Geometry check sheet. Reference: the model listing, model coordinates, mm. Give positions to 0.01 mm unless a question says otherwise; leave off trailing zeros. Write each loop counter-clockwise with the first axis right and the second up, starting at its lowest first coordinate (ties: lowest second). Pieces come first, ordered by that corner, then holes. Notation, with made-up numbers: (1.25, 84.25) -> (23.25, 84.25) arc R19 cw to (23.25, 121.25) -> close; hole circle Ø10 at (2.5, 10.5). An arc over 180 degrees is marked (long way). Write item = value, one per line. Start each with the question number.
1. Thickness scan on line 1 along Z through (x, y) = (27, 96.5); line 2 along X through (y, z) = (48, -7); line 3 along Y through (x, z) = (1, -5). Record the ranges inside material, lowest first.
2. Cross-section at C-C, the plane z = -7.75. Record the cut outline in (x, y) (3 decimals), plus the area to 3 significant figures.
3. Cross-section at B-B, the plane y = 13. Record the cut outline in (x, z), plus the area to 3 significant figures.
4. Cross-section at A-A, the plane x = 59. Record the cut outline in (y, z) (3 decimals).
5. Depth check by flat-ended pin: P1, Ø5, axis at x = 12, z = -10, coming from the +Y side; P2, Ø2.5, axis at x = -11.5, z = -7.5, coming from the +Y side (3 decimals). Enter the tip coordinate at first touch or a pass-through.
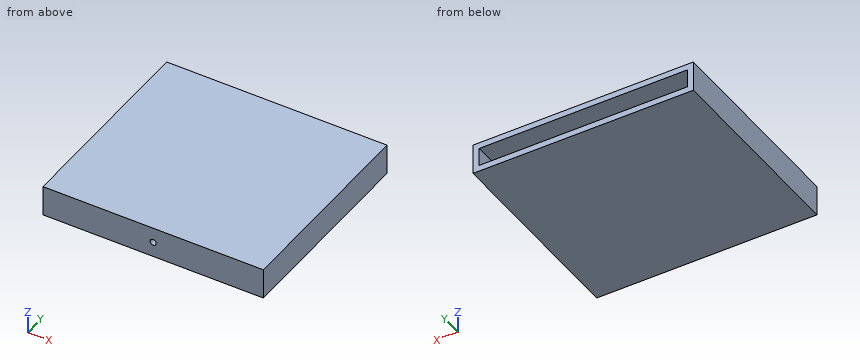
Autodesk Inventor part; units mm, degrees
ref_plane "YZ Plane" through (0, 0, 0) normal (1, 0, 0) x (0, 1, 0)
ref_plane "XZ Plane" through (0, 0, 0) normal (0, 1, 0) x (-1, 0, 0)
ref_plane "XY Plane" through (0, 0, 0) normal (0, 0, 1) x (1, 0, 0)
sketch "Sketch1" plane through (0, 0, 0) normal (0, 1, 0) x (-1, 0, 0)
  line L0 (43.1683, -15.7294) -> (-71.1317, -15.7294)
  line L1 (-71.1317, -15.7294) -> (-71.1317, 0.1456)
  line L2 (-71.1317, 0.1456) -> (43.1683, 0.1456)
  line L3 (43.1683, 0.1456) -> (43.1683, -15.7294)
  point P0 (0, 0)
  dimension "d0" = 114.3
  dimension "d1" = 15.875
extrude "Extrusion1" add sketch "Sketch1" along normal blind 3.175
sketch "Sketch6" plane through (0, 3.175, 0) normal (0, 1, 0) x (1, 0, 0)
  line L0 (71.1317, 15.7294) -> (-43.1683, 15.7294)
  line L1 (-43.1683, 15.7294) -> (71.1317, 15.7294)
  line L2 (71.1317, 15.7294) -> (71.1317, 12.5544)
  line L3 (71.1317, 12.5544) -> (-43.1683, 12.5544)
  line L4 (-43.1683, 12.5544) -> (-43.1683, 15.7294)
  point P0 (0, 0)
  dimension "d33" = 3.175
  dimension "d34" = 114.3
extrude "Extrusion2" add sketch "Sketch6" along normal blind 101.6
sketch "Sketch9" plane through (0, 3.175, 0) normal (0, 1, 0) x (1, 0, 0)
  line L0 (-43.1683, -0.1456) -> (71.1317, -0.1456)
  line L1 (-43.1683, -0.1456) -> (71.1317, -0.1456)
  line L2 (71.1317, -0.1456) -> (71.1317, 3.0294)
  line L3 (71.1317, 3.0294) -> (-43.1683, 3.0294)
  line L4 (-43.1683, 3.0294) -> (-43.1683, -0.1456)
  point P0 (0, 0)
  dimension "d41" = 3.175
  dimension "d42" = 114.3
extrude "Extrusion3" add sketch "Sketch9" along normal blind 101.6
sketch "Sketch11" plane through (0, 3.175, 0) normal (0, 1, 0) x (1, 0, 0)
  line L0 (-43.1683, 12.5544) -> (71.1317, 12.5544)
  line L1 (-43.1683, 12.5544) -> (-39.9933, 12.5544)
  line L2 (-39.9933, 12.5544) -> (-39.9933, 3.0294)
  line L3 (-39.9933, 3.0294) -> (-43.1683, 3.0294)
  line L4 (-43.1683, 3.0294) -> (-43.1683, 12.5544)
  point P0 (0, 0)
  dimension "d45" = 3.175
  dimension "d46" = 9.525
extrude "Extrusion4" add sketch "Sketch11" along normal blind 101.6
sketch "Sketch13" plane through (0, 3.175, 0) normal (0, 1, 0) x (1, 0, 0)
  line L0 (71.1317, 12.5544) -> (-39.9933, 12.5544)
  line L1 (71.1317, 12.5544) -> (67.9567, 12.5544)
  line L2 (67.9567, 12.5544) -> (67.9567, 3.0294)
  line L3 (67.9567, 3.0294) -> (71.1317, 3.0294)
  line L4 (71.1317, 3.0294) -> (71.1317, 12.5544)
  point P0 (0, 0)
  dimension "d51" = 3.175
  dimension "d52" = 9.525
extrude "Extrusion5" add sketch "Sketch13" along normal blind 101.6
sketch "Sketch14" plane through (0, 3.175, 0) normal (0, 1, 0) x (1, 0, 0)
  line L0 (67.9567, 12.5544) -> (-39.9933, 12.5544)
  line L1 (-39.9933, 12.5544) -> (67.9567, 12.5544)
  line L2 (67.9567, 12.5544) -> (67.9567, 9.3794)
  line L3 (67.9567, 9.3794) -> (-39.9933, 9.3794)
  line L4 (-39.9933, 9.3794) -> (-39.9933, 12.5544)
  point P0 (0, 0)
  dimension "d55" = 3.175
  dimension "d56" = 107.95
extrude "Extrusion6" add sketch "Sketch14" along normal blind 3.175
sketch "Sketch15" plane through (0, 3.175, 0) normal (0, 1, 0) x (1, 0, 0)
  line L0 (67.9567, 3.0294) -> (-39.9933, 3.0294)
  line L1 (-39.9933, 3.0294) -> (67.9567, 3.0294)
  line L2 (67.9567, 3.0294) -> (67.9567, 6.2044)
  line L3 (67.9567, 6.2044) -> (-39.9933, 6.2044)
  line L4 (-39.9933, 6.2044) -> (-39.9933, 3.0294)
  point P0 (0, 0)
  dimension "d59" = 3.175
  dimension "d60" = 107.95
extrude "Extrusion7" add sketch "Sketch15" along normal blind 3.175
sketch "Sketch17" plane through (0, 3.175, 0) normal (0, 1, 0) x (1, 0, 0)
  line L0 (67.9567, 9.3794) -> (-39.9933, 9.3794)
  line L1 (-39.9933, 9.3794) -> (-36.8183, 9.3794)
  line L2 (-36.8183, 9.3794) -> (-36.8183, 6.2044)
  line L3 (-36.8183, 6.2044) -> (-39.9933, 6.2044)
  line L4 (-39.9933, 6.2044) -> (-39.9933, 9.3794)
  point P0 (0, 0)
  dimension "d64" = 3.175
  dimension "d65" = 3.175
extrude "Extrusion8" add sketch "Sketch17" along normal blind 3.175
sketch "Sketch18" plane through (0, 3.175, 0) normal (0, 1, 0) x (1, 0, 0)
  line L0 (-36.8183, 9.3794) -> (67.9567, 9.3794)
  line L1 (67.9567, 9.3794) -> (64.7817, 9.3794)
  line L2 (64.7817, 9.3794) -> (64.7817, 6.2044)
  line L3 (64.7817, 6.2044) -> (67.9567, 6.2044)
  line L4 (67.9567, 6.2044) -> (67.9567, 9.3794)
  point P0 (0, 0)
  dimension "d68" = 3.175
  dimension "d69" = 3.175
extrude "Extrusion9" add sketch "Sketch18" along normal blind 3.175
sketch "Sketch20" plane through (0, 104.775, 0) normal (0, 1, 0) x (1, 0, 0)
  line L0 (-43.1683, -0.1456) -> (71.1317, -0.1456)
  line L1 (-43.1683, -0.1456) -> (-43.1683, 7.7919)
  line L2 (-43.1683, 15.7294) -> (-43.1683, -0.1456)
  line L3 (-43.1683, 7.7919) -> (13.9817, 7.7919)
  point P0 (0, 0)
  dimension "d79" = 7.9375
  dimension "d80" = 57.15
hole "Hole6" at (13.9817, 104.775, -7.7919) direction (0, -1, 0) diameter 3.175 end through all
properties part number "sing_cell_bottom_case_alternate"
Answers:
q1.line_1 = -15.73 to -12.55, -3.03 to 0.15
q1.line_2 = -43.17 to -39.99, 67.96 to 71.13
q1.line_3 = 0 to 6.35
q2.outline = (-43.168, 0) -> (12.395, 0) -> (12.395, 3.175) -> (-36.818, 3.175) -> (-36.818, 6.35) -> (-39.993, 6.35) -> (-39.993, 104.775) -> (-43.168, 104.775) -> close; (15.569, 0) -> (71.132, 0) -> (71.132, 104.775) -> (67.957, 104.775) -> (67.957, 6.35) -> (64.782, 6.35) -> (64.782, 3.175) -> (15.569, 3.175) -> close
q2.area = 1,020 mm^2
q3.outline = (-43.17, -15.73) -> (71.13, -15.73) -> (71.13, 0.15) -> (-43.17, 0.15) -> close; hole (-39.99, -12.55) -> (67.96, -12.55) -> (67.96, -3.03) -> (-39.99, -3.03) -> close
q3.area = 786 mm^2
q4.outline = (0, -15.729) -> (104.775, -15.729) -> (104.775, -12.554) -> (6.35, -12.554) -> (6.35, -9.379) -> (3.175, -9.379) -> (3.175, -6.204) -> (6.35, -6.204) -> (6.35, -3.029) -> (104.775, -3.029) -> (104.775, 0.146) -> (0, 0.146) -> close
q5.P1 = 6.35
q5.P2 = 3.175
